Here's how the part is built. I have some questions about the finished solid (model axes, mm). A direction names the side the tool comes from. Round coordinates to 2 decimals unless told otherwise and drop trailing zeros. Order: outer loops, then holes, each group sorted by start corner. A loop starts at its lowest first (then second) coordinate and runs counter-clockwise, first axis right, second up. Notation, with made-up numbers: (68, 54.5) -> (81, 54.5) arc R28 ccw to (81, 87.5) -> close; hole circle Ø10 at (-10, 35). An arc over 180 degrees is marked (long way). One line per item, written item: value.
```python
from build123d import *
from build123d.topology import SkipClean

# Parameters (mm, degrees)
SKETCH2_W           = 6.5
SKETCH2_H           = 5
SKETCH2_W_2         = 4.5
SKETCH2_H_2         = 4.5
BOSS_EXTRUDE1_DEPTH = 2
BOSS_EXTRUDE2_START = 2
SKETCH2_2_W         = 6.5
SKETCH2_2_H         = 5
SKETCH2_2_W_2       = 4.5
SKETCH2_2_H_2       = 4.5
BOSS_EXTRUDE2_DEPTH = 38
BOSS_EXTRUDE3_DEPTH = 3
SKETCH6_R           = 2.6
BOSS_EXTRUDE4_DEPTH = 5


with BuildPart() as part:
    # Sketch2 → Boss-Extrude1 (new body)
    with BuildSketch(Plane(origin=(0, 0, 0), x_dir=(0, 0, -1), z_dir=(1, 0, 0))):
        Rectangle(SKETCH2_W, SKETCH2_H)
        Rectangle(SKETCH2_W_2, SKETCH2_H_2, mode=Mode.SUBTRACT)
    extrude(amount=BOSS_EXTRUDE1_DEPTH)

    # Sketch2<2> → Boss-Extrude2 (add)
    with BuildSketch(Plane(origin=(0, 0, 0), x_dir=(0, 0, -1), z_dir=(1, 0, 0)).offset(BOSS_EXTRUDE2_START)):
        Rectangle(SKETCH2_2_W, SKETCH2_2_H)
        Rectangle(SKETCH2_2_W_2, SKETCH2_2_H_2, mode=Mode.SUBTRACT)
        Rectangle(SKETCH2_2_W_2, SKETCH2_2_H_2)
    extrude(amount=BOSS_EXTRUDE2_DEPTH)

    # Sketch5 → Boss-Extrude3 (add)
    with BuildSketch(Plane(origin=(40, 0, 0), x_dir=(0, 0, -1), z_dir=(1, 0, 0))):
        with BuildLine():
            Line((-5.992134655, -1.935858048), (-3.25, 2.5))
            Line((-3.25, 2.5), (3.25, 2.5))
            Line((3.25, 2.5), (3.25, -2.5))
            Line((3.25, -2.5), (0, -2.5))
            Line((0, -2.5), (-1.669999982, -4.821353165))
            ThreePointArc((-1.669999982, -4.821353165), (-5.224212214, -5.465373947), (-5.992134655, -1.935858048))
        make_face()
    extrude(amount=BOSS_EXTRUDE3_DEPTH)

    # Sketch6 → Boss-Extrude4 (add)
    with SkipClean():  # the faces are left unmerged after this step: merging them gives an invalid solid
        with BuildSketch(Plane(origin=(43, 0, 0), x_dir=(0, 0, -1), z_dir=(1, 0, 0))):
            with Locations(Location((-3.780581608, -3.302983909, 0), (0, 0, 148.276697379))):
                Circle(SKETCH6_R)
        extrude(amount=BOSS_EXTRUDE4_DEPTH)


solid = part.part
```
Q1. I want a section at D-D on y = -3. Write out the boundary of the cut face in (x, z), then the cut area to 3 significant figures.
Answers:
outline: (40, 0.36) -> (43, 0.36) -> (43, 1.2) -> (48, 1.2) -> (48, 6.36) -> (40, 6.36) -> close
area: 43.8 mm2
Q2. For P1, Ø2, axis at y = 0.5, z = 0.5, coming from the +X side; P2, Ø1.5, axis at x = 21, y = -0.5, coming from the +Z side; P3, Ø5, axis at y = -0.5, z = 1, coming from the -X side; P4, Ø1, axis at x = 0.5, z = 1, coming from the -Y side, each with a flat end and sliding along its axis, tell me the tip position at first contact or that it passes through.
Answers:
P1: x = 43
P2: z = 3.25
P3: x = 0
P4: y = -2.5
Q3. I want a section at A-A on z = -1.5. Write out the boundary of the cut face in (x, y), then the cut area to 3 significant figures.
Answers:
outline: (0, -2.5) -> (43, -2.5) -> (43, 2.5) -> (0, 2.5) -> (0, 2.25) -> (2, 2.25) -> (2, -2.25) -> (0, -2.25) -> close
area: 206 mm2
Q4. If we mould it in two halves opening along Z, with no side actions, what happens to faces 4 (the face through (41.48, -3.64, 0.82)), 5 (the face through (48, -3, 4)), 6 (the face through (1, 0, 2.25)), 7 (the face through (1, 2.25, 0))? For each: pulls with the +Z half, pulls with the -Z half, needs draft (parallel to the pull), parting line crosses it, or undercut.
Answers:
face 4: pulls with the -Z half
face 5: needs draft
face 6: undercut
face 7: undercut
Q5. I need wall thicknesses on line 1 along Z through (x, y) = (4.5, -1.75); line 2 along Y through (x, z) = (13, -1.75); line 3 along X through (y, z) = (-2, 4). Which ranges of each line are inside material? Lowest first, please.
Answers:
line 1: -3.25 to 3.25
line 2: -2.5 to 2.5
line 3: 40 to 48
Q6. I want a section at C-C on x = 43.5. Write out the boundary of the cut face in (y, z).
Answers:
outline: circle Ø5.2 at (-3.3, 3.78)
Q7. I want a section at B-B on y = -0.25. Write out the boundary of the cut face in (x, z), then the cut area to 3 significant figures.
Answers:
outline: (0, -3.25) -> (43, -3.25) -> (43, 4.95) -> (40, 4.95) -> (40, 3.25) -> (0, 3.25) -> (0, 2.25) -> (2, 2.25) -> (2, -2.25) -> (0, -2.25) -> close
area: 276 mm2
Q8. Which directions (+Z, -Z, +X, -X, +Y, -Y) give clear straight access to the entire face, cutting with the end or side of a thin tool? Please do faces 1 (the face through (1, 0, -2.25)), 2 (the face through (20, 0, 3.25)), 3 (the face through (0, -0.17, 2.42)).
Answers:
face 1: -X
face 2: +Z, -X, +Y, -Y
face 3: +Z, -Z, -X, +Y, -Y
